Source: CAD feature listing. Evaluate the final solid. Frame: model axes, mm. A direction names the side the tool comes from. Round coordinates to 2 decimals unless told otherwise and drop trailing zeros. Loops run counter-clockwise (first coordinate to the right, second up) from the corner with the lowest first, then second, coordinate; pieces in that order, holes last.
Item 1: Section query B-B on y = -27. Return loops of the section in (x, z), then the cut area to 3 significant figures.
Item 2: First-contact query: P1, Ø4, axis at x = 35.5, y = -31.5, coming from the -Z side; P2, Ø1, axis at x = 60.5, y = -9, coming from the +Z side; P3, Ø5.5, axis at x = 59, y = -46.5, coming from the +Z side. Flat tips, straight axial feed; report the tip coordinate or a pass-through.
Item 3: Section query A-A on x = 5.5. Return loops of the section in (y, z), then the cut area to 3 significant figures.
Item 4: Ray query, L1, parallel to X at y = -31.5, z = 2.25; L2, parallel to Z at x = 16, y = -13; L3, parallel to X at y = -5.5, z = 23.25. Return the intervals inside material, ascending.
Item 5: Section query C-C on x = 47.5. Return loops of the section in (y, z).
Item 6: Access query for faces 1 (the flat face through (59, -46, 15)), 2 (the flat face through (4, -24.84, 18)), 3 (the flat face through (32, -25, 3)), 4 (the flat face through (0, -25, 8)). Directions: +Z, -Z, +X, -X, +Y, -Y. A direction counts if a zero-diameter tool reaches every point of the face in a straight line with its end or side. Return the directions, or none.
Item 7: Pull-direction query (Y, two-part tool) for faces 5 (the flat face through (59, -9.56, 18)), 6 (the flat face through (31, 0, 15)), 7 (the flat face through (5, -50, 21)); classes: released by +Y, released by -Y, zero draft, split by the parting line, or undercut.
```python
from build123d import *

# Parameters (mm, degrees)
F1_DEPTH = 51
F2_W     = 9
F2_H     = 7
F3_DEPTH = 6


with BuildPart() as f1:
    # F0 (on Front) → F1 (new body)
    with BuildSketch(Plane.XZ):
        Polygon((0, 21), (0, 0), (14.25, 0), (14.25, 3), (49.25, 3), (49.25, 0), (63.5, 0), (63.5, 21), (54.5, 21), (54.5, 30), (9, 30), (9, 21), align=None)
    extrude(amount=F1_DEPTH)

    # F2 (on face) → F3 (cut)
    with BuildSketch(Plane.XY.offset(21)):
        with Locations((59, -4.78)):
            Rectangle(F2_W, F2_H)
        with Locations((59, -13.06)):
            Rectangle(F2_W, F2_H)
        with Locations((59, -21.34)):
            Rectangle(F2_W, F2_H)
        with Locations((59, -29.62)):
            Rectangle(F2_W, F2_H)
        with Locations((59, -37.9)):
            Rectangle(F2_W, F2_H)
        with Locations((59, -46.18)):
            Rectangle(F2_W, F2_H)
        with Locations((4.5, -4.78)):
            Rectangle(F2_W, F2_H)
        with Locations((4.5, -13.06)):
            Rectangle(F2_W, F2_H)
        with Locations((4.5, -21.34)):
            Rectangle(F2_W, F2_H)
        with Locations((4.5, -29.62)):
            Rectangle(F2_W, F2_H)
        with Locations((4.5, -37.9)):
            Rectangle(F2_W, F2_H)
        with Locations((4.5, -46.18)):
            Rectangle(F2_W, F2_H)
    extrude(amount=-F3_DEPTH, mode=Mode.SUBTRACT)


solid = f1.part
```
Data:
1. outline: (0, 0) - (14.25, 0) - (14.25, 3) - (49.25, 3) - (49.25, 0) - (63.5, 0) - (63.5, 15) - (54.5, 15) - (54.5, 30) - (9, 30) - (9, 15) - (0, 15) - close
1. area: 1,530 mm2
2. P1: stops at z = 3
2. P2: stops at z = 21
2. P3: stops at z = 15
3. outline: (-51, 0) - (0, 0) - (0, 21) - (-1.28, 21) - (-1.28, 15) - (-8.28, 15) - (-8.28, 21) - (-9.56, 21) - (-9.56, 15) - (-16.56, 15) - (-16.56, 21) - (-17.84, 21) - (-17.84, 15) - (-24.84, 15) - (-24.84, 21) - (-26.12, 21) - (-26.12, 15) - (-33.12, 15) - (-33.12, 21) - (-34.4, 21) - (-34.4, 15) - (-41.4, 15) - (-41.4, 21) - (-42.68, 21) - (-42.68, 15) - (-49.68, 15) - (-49.68, 21) - (-51, 21) - close
3. area: 819 mm2
4. L1: x = 0 to 14.25, 49.25 to 63.5
4. L2: z = 3 to 30
4. L3: x = 9 to 54.5
5. outline: (-51, 3) - (0, 3) - (0, 30) - (-51, 30) - close
6. face 1: +Z, +X
6. face 2: +Z, -X
6. face 3: -Z, +Y, -Y
6. face 4: +Z, -Z, -X, +Y, -Y
7. face 5: undercut
7. face 6: released by +Y
7. face 7: zero draft
